Read the model definition and answer for the solid it produces. Units are mm, in the model's axes. Coordinates: 2 decimals unless noted, no trailing zeros. Write each loop counter-clockwise with the first axis right and the second up, starting at its lowest first coordinate (ties: lowest second). Pieces come first, ordered by that corner, then holes.
(1) Given pin 1 (1 mm diameter, centred on y = 156, z = 0.5, fed in from -X), flat-ended and moving along its own axis, determine where the tip first touches the part or whether it passes through.
(2) The part is cut by section C-C, the plane x = 107. Determine the outline of the cut face in (y, z).
(3) The part is cut by section B-B, the plane z = 0.2. Determine the outline of the cut face in (x, y).
(4) Straight lines are drawn through the part: line 1 along Y through (x, z) = (113, 1); line 2 along Y through (x, z) = (52.5, 0.8); line 3 along Y through (x, z) = (72, -0.3). For each, find the intervals that lie inside material, in ascending order.
(5) The part is cut by section D-D, the plane y = 14. Determine the outline of the cut face in (x, z).
(6) Determine the mould class of faces 1 (the cylindrical face through (138.412, 24.053, 0.022)), 2 (the cylindrical face through (123.16, 19.14, 0.02)), 3 (the flat face through (120, 53, 1.588)), 4 (the cylindrical face through (69.28, 141.69, 0.02)) for opening direction Y: pulls with the +Y half, pulls with the -Y half, needs draft (parallel to the pull), parting line crosses it, or undercut.
(7) The part is cut by section A-A, the plane x = 45.5. Determine the outline of the cut face in (y, z).
```python
from build123d import *

# Parameters (mm, degrees)
BOSS_EXTRUDE1_DEPTH = 1.5875
CUT_EXTRUDE1_DEPTH  = 3.175
FILLET1_R           = 8.89
SKETCH4_W           = 218.524279389
SKETCH4_H           = 440.65456999
CUT_EXTRUDE3_DEPTH  = 139.43
CUT_EXTRUDE4_DEPTH  = 4.175


with BuildPart() as part:
    # Sketch1 → Boss-Extrude1 (new body, symmetric)
    with BuildSketch(Plane.XY):
        with BuildLine():
            Line((-127.293308919, -32.555250036), (-85.984130762, -73.864428193))
            Line((-85.984130762, -73.864428193), (-85.984130762, -86.643760402))
            ThreePointArc((-85.984130762, -86.643760402), (-70.818680903, -97.099597285), (-54.399250036, -105.449308919))
            ThreePointArc((-54.399250036, -105.449308919), (97.88479172, 119.72879172), (-127.293308919, -32.555250036))
        make_face()
    extrude(amount=BOSS_EXTRUDE1_DEPTH, both=True)

    # Sketch2 → Cut-Extrude1 (cut)
    with BuildSketch(Plane.XY.offset(1.5875)):
        with BuildLine():
            Line((-114.372852664, -23.923091601), (-70.744130762, -67.551813503))
            Line((-70.744130762, -67.551813503), (-70.744130762, -79.00759425))
            ThreePointArc((-70.744130762, -79.00759425), (96.569405073, 98.330117066), (-114.372852664, -23.923091601))
        make_face()
    extrude(amount=-CUT_EXTRUDE1_DEPTH, mode=Mode.SUBTRACT)

    # Fillet1
    fillet1_edges = [part.edges().sort_by_distance(p)[0] for p in [
        (-114.372852664, -23.923091601, 0),
        (-70.744130762, -79.00759425, 0),
        (-70.744130762, -67.551813503, 0),
        (-85.984130762, -86.643760402, -0.79375),
        (-85.984130762, -73.864428193, -0.79375),
        (-127.293308919, -32.555250036, -0.79375),
    ]]
    fillet(fillet1_edges, radius=FILLET1_R)

    # Sketch4 → Cut-Extrude3 (cut, through all)
    with BuildSketch(Plane(origin=(0, 0, 0), x_dir=(0, 0, -1), z_dir=(1, 0, 0))):
        with Locations((12.98164036, 12.468370851)):
            Rectangle(SKETCH4_W, SKETCH4_H)
    extrude(amount=-CUT_EXTRUDE3_DEPTH, mode=Mode.SUBTRACT)

    # Sketch5 → Cut-Extrude4 (cut, through all)
    with BuildSketch(Plane(origin=(0, 0, -1.5875), x_dir=(-1, 0, 0), z_dir=(0, 0, -1))):
        with BuildLine():
            Line((-114.517752975, -38.815428837), (-122.170481647, -43.250072804))
            ThreePointArc((-122.170481647, -43.250072804), (-121.36689626, -44.736337881), (-120.545230584, -46.212684341))
            Line((-120.545230584, -46.212684341), (-112.823974718, -41.738329871))
            Line((-112.823974718, -41.738329871), (-114.517752975, -38.815428837))
        make_face()
        with BuildLine():
            Line((-109.598496198, 91.009030044), (-117.267867629, 95.404261839))
            ThreePointArc((-117.267867629, 95.404261839), (-118.157043978, 93.967351685), (-119.028614444, 92.519694857))
            Line((-119.028614444, 92.519694857), (-111.278220029, 88.078029687))
            Line((-111.278220029, 88.078029687), (-109.598496198, 91.009030044))
        make_face()
        with BuildLine():
            Line((-3.302, 160.234612745), (-3.302, 151.384))
            Line((-3.302, 151.384), (0, 151.384))
            Line((0, 151.384), (0, 160.274))
            ThreePointArc((0, 160.274), (-1.651117452, 160.264152836), (-3.302, 160.234612745))
        make_face()
        with BuildLine():
            Line((-3.302, -107.696), (-3.302, -116.546612745))
            ThreePointArc((-3.302, -116.546612745), (-1.651117452, -116.576152836), (0, -116.586))
            Line((0, -116.586), (0, -107.696))
            Line((0, -107.696), (-3.302, -107.696))
        make_face()
    extrude(amount=-CUT_EXTRUDE4_DEPTH, mode=Mode.SUBTRACT)


solid = part.part
```
Computed:
1. pin 1: stops at x = 3.3
2. outline: (-65.98, -1.59) - (-39.2, -1.59) - (-39.2, 1.59) - (-65.98, 1.59) - close; (82.89, -1.59) - (109.67, -1.59) - (109.67, 1.59) - (82.89, 1.59) - close
3. outline: (0, -107.7) - (3.3, -107.7) - (3.3, -116.55) arc R138.43 ccw to (120.55, -46.21) - (112.82, -41.74) - (114.52, -38.82) - (122.17, -43.25) arc R138.43 ccw to (119.03, 92.52) - (111.28, 88.08) - (109.6, 91.01) - (117.27, 95.4) arc R138.43 ccw to (3.3, 160.23) - (3.3, 151.38) - (0, 151.38) - (0, 145.03) arc R123.19 cw to (0, -101.35) - close
4. line 1: y = -58.12 to -41.84, -41.43 to -27.21, 70.9 to 89.06, 92.96 to 101.81
4. line 2: y = -106.24 to -89.6, 133.29 to 149.93
4. line 3: y = -96.39 to -78.11, 121.8 to 140.08
5. outline: (122.94, -1.59) - (138.21, -1.59) - (138.21, 1.59) - (122.94, 1.59) - close
6. face 1: parting line crosses it
6. face 2: undercut
6. face 3: needs draft
6. face 4: pulls with the +Y half
7. outline: (-108.89, -1.59) - (-92.64, -1.59) - (-92.64, 1.59) - (-108.89, 1.59) - close; (136.32, -1.59) - (152.58, -1.59) - (152.58, 1.59) - (136.32, 1.59) - close
